from build123d import *

# Parameters (mm, degrees)
F1_DEPTH = 76.2
F3_DEPTH = 101.6
F5_DEPTH = 25.4
F7_DEPTH = 25.4


with BuildPart() as f1:
    # F0 (on Front) → F1 (new body)
    with BuildSketch(Plane.XZ):
        Polygon((-75.980723, 12.7), (-75.980723, 0), (-37.880723, 0), (-37.880723, 12.7), (-50.580723, 12.7), align=None)
        Polygon((-50.580723, 12.7), (-37.880723, 12.7), (38.319277, 12.7), (51.019277, 12.7), (51.019277, 50.8), (-50.580723, 50.8), align=None)
        Polygon((51.019277, 12.7), (38.319277, 12.7), (38.319277, 0), (76.419277, 0), (76.419277, 12.7), align=None)
    extrude(amount=F1_DEPTH)

    # F2 (on face) → F3 (cut)
    with BuildSketch(Plane.YZ.offset(51.019277)):
        Polygon((-38.1, 50.8), (-50.8, 50.8), (-38.1, 38.1), align=None)
        Polygon((-38.1, 50.8), (-38.1, 38.1), (-25.4, 50.8), align=None)
    extrude(amount=-F3_DEPTH, mode=Mode.SUBTRACT)

    # F4 (on face) → F5 (cut)
    with BuildSketch(Plane.XY.offset(12.7)):
        Polygon((51.019277, -25.4), (51.019277, -50.8), (76.419277, -76.2), (76.419277, 0), align=None)
    extrude(amount=-F5_DEPTH, mode=Mode.SUBTRACT)

    # F6 (on face) → F7 (cut)
    with BuildSketch(Plane.XY.offset(12.7)):
        Polygon((-50.580723, -50.8), (-50.580723, -25.4), (-75.980723, 0), (-75.980723, -76.2), align=None)
    extrude(amount=-F7_DEPTH, mode=Mode.SUBTRACT)


solid = f1.part
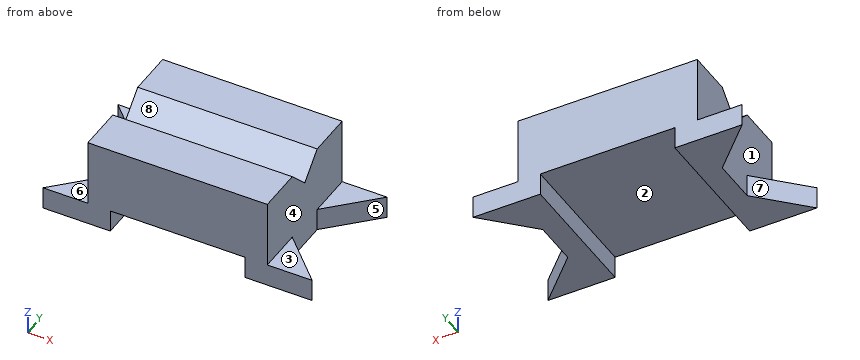
Read the model definition and answer for the solid it produces. Units are mm, in the model's axes. Face numbers are marked on the shaded views. A direction names the side the tool comes from. Give positions to 0.01 mm unless a question says otherwise; leave off trailing zeros. Write each loop counter-clockwise with the first axis right and the second up, starting at its lowest first coordinate (ties: lowest second). Pieces come first, ordered by that corner, then holes. Notation, with made-up numbers: (10.25, 74.25) - (26.25, 74.25) arc R24 cw to (26.25, 111.25) - close; hole circle Ø3 at (-11.75, 68.5). An arc over 180 degrees is marked (long way). Use CSV: the item, a comma, the result in double quotes. Start each with the question number.
Item 1: For the marked faces 5, 6, 7 and 8, determine the directions among +Z, -Z, +X, -X, +Y, -Y from which every point of the face is accessible in a straight line to the end or side of a thin tool.
Item 2: The part is cut by section B-B, the plane y = -27.5. Give the vertices of the cut face in (x, z), and give its area (3 significant figures).
Item 3: The mould has two halves that part along X. Classify the marked faces 1, 2, 3 and 4: pulls with the +X half, pulls with the -X half, needs draft (parallel to the pull), parting line crosses it, or undercut.
Item 4: The part is cut by section D-D, the plane x = -9. Give the vertices of the cut face in (y, z), and give its area (3 significant figures).
Item 5: The part is cut by section A-A, the plane z = 9.5. Give the vertices of the cut face in (x, y), and give its area (3 significant figures).
Item 6: Consider line 1 (X direction, y = -47.5, z = 4.5); line 2 (X direction, y = -24.5, z = 34); line 3 (Z direction, x = 22.5, y = -18.5). Determine where each line is inside the solid, lowest interval first.
Item 7: Flat-ended cylindrical pins translate along their axes: P1, Ø12.5, axis at x = -62, y = -66.5, coming from the +Z side; P2, Ø4, axis at x = 51, y = -33.5, coming from the +Z side; P3, Ø2, axis at y = -53.5, z = 25.5, coming from the +X side. Find the tip coordinate at first contact, or state that the pin passes through.
Item 8: The part is cut by section C-C, the plane x = -54.5. Give the vertices of the cut face in (y, z), and give its area (3 significant figures).
Taken from the geometry:
1,face 5,"+Z, -Z, +X"
1,face 6,"+Z, -X, +Y, -Y"
1,face 7,"+Z, -Z, -X"
1,face 8,"+Z, +X, -X"
2,outline,"(-50.58, 0) - (-37.88, 0) - (-37.88, 12.7) - (38.32, 12.7) - (38.32, 0) - (51.02, 0) - (51.02, 48.7) - (-50.58, 48.7) - close"
2,area,"3,980 mm2"
3,face 1,"pulls with the -X half"
3,face 2,"undercut"
3,face 3,"needs draft"
3,face 4,"pulls with the +X half"
4,outline,"(-76.2, 12.7) - (0, 12.7) - (0, 50.8) - (-25.4, 50.8) - (-38.1, 38.1) - (-50.8, 50.8) - (-76.2, 50.8) - close"
4,area,"2,740 mm2"
5,outline,"(-75.98, -76.2) - (-37.88, -76.2) - (-37.88, 0) - (-75.98, 0) - (-50.58, -25.4) - (-50.58, -50.8) - close; (38.32, -76.2) - (76.42, -76.2) - (51.02, -50.8) - (51.02, -25.4) - (76.42, 0) - (38.32, 0) - close"
5,area,"3,230 mm2"
6,line 1,"-50.58 to -37.88, 38.32 to 51.02"
6,line 2,"-50.58 to 51.02"
6,line 3,"12.7 to 50.8"
7,P1,"z = 12.7"
7,P2,"z = 44.7"
7,P3,"x = 51.02"
8,outline,"(-76.2, 0) - (-54.72, 0) - (-54.72, 12.7) - (-76.2, 12.7) - close; (-21.48, 0) - (0, 0) - (0, 12.7) - (-21.48, 12.7) - close"
8,area,"546 mm2"
